Input: part model. Units: mm. Frame: model coordinates. A direction names the side the tool comes from. Give positions to 0.01 mm unless a question says otherwise; leave off trailing zeros. Order: outer loops, then holes, each group sorted by start corner. A loop starts at its lowest first (then second) coordinate and runs counter-clockwise, first axis right, second up. Notation, with made-up numbers: (27.5, -15) -> (43.5, -15) arc R28 cw to (43.5, 3) -> close; hole circle Ø11 at (18, 38). An arc over 180 degrees is marked (long way). Use a Markdown table: item, result. Add a question column.
from build123d import *

# Parameters (mm, degrees)
BOSS_EXTRUDE1_DEPTH = 2
SKETCH3_W           = 2
SKETCH3_H           = 40
SKETCH3_W_2         = 30
SKETCH3_H_2         = 2
BOSS_EXTRUDE2_DEPTH = 3
SKETCH4_R           = 1.75
CUT_EXTRUDE1_DEPTH  = 3
CHAMFER1_SIZE       = 1


with BuildPart() as part:
    # Sketch1 → Boss-Extrude1 (new body)
    with BuildSketch(Plane.XY):
        with BuildLine():
            Line((65.230528188, -85.753133266), (65.230528188, -22.753132266))
            ThreePointArc((65.230528188, -22.753132266), (64.351848531, -20.631811922), (62.230528188, -19.753132266))
            Line((62.230528188, -19.753132266), (-24.769470492, -19.753132266))
            ThreePointArc((-24.769470492, -19.753132266), (-26.890790836, -20.631811922), (-27.769470492, -22.753132266))
            Line((-27.769470492, -22.753132266), (-27.769470492, -85.753133266))
            ThreePointArc((-27.769470492, -85.753133266), (-26.890790836, -87.874453609), (-24.769470492, -88.753133266))
            Line((-24.769470492, -88.753133266), (62.230528188, -88.753133266))
            ThreePointArc((62.230528188, -88.753133266), (64.351848531, -87.874453609), (65.230528188, -85.753133266))
        make_face()
    extrude(amount=BOSS_EXTRUDE1_DEPTH)

    # Sketch3 → Boss-Extrude2 (add)
    with BuildSketch(Plane(origin=(0, 0, 0), x_dir=(-1, 0, 0), z_dir=(0, 0, -1))):
        with Locations((-61.930528188, -54.253132766)):
            Rectangle(SKETCH3_W, SKETCH3_H)
        with Locations((24.469470492, -54.253132766)):
            Rectangle(SKETCH3_W, SKETCH3_H)
        with Locations((-18.730528848, -23.053132266)):
            Rectangle(SKETCH3_W_2, SKETCH3_H_2)
        with Locations((-18.730528848, -85.453133266)):
            Rectangle(SKETCH3_W_2, SKETCH3_H_2)
    extrude(amount=BOSS_EXTRUDE2_DEPTH)

    # Sketch4 → Cut-Extrude1 (cut)
    with BuildSketch(Plane(origin=(0, 0, 0), x_dir=(-1, 0, 0), z_dir=(0, 0, -1))):
        with Locations((-59.230528188, -25.753132266)):
            Circle(SKETCH4_R)
        with Locations((21.769470706, -25.703133912)):
            Circle(SKETCH4_R)
        with Locations((21.769470492, -82.753133266)):
            Circle(SKETCH4_R)
        with Locations((-59.230528188, -82.753133266)):
            Circle(SKETCH4_R)
    extrude(amount=-CUT_EXTRUDE1_DEPTH, mode=Mode.SUBTRACT)

    # Chamfer1
    chamfer1_edges = [part.edges().sort_by_distance(p)[0] for p in [
        (60.980528188, -82.753133266, 2),
        (-20.019470492, -82.753133266, 2),
        (-20.019470706, -25.703133912, 2),
        (60.980528188, -25.753132266, 2),
    ]]
    chamfer(chamfer1_edges, length=CHAMFER1_SIZE)


solid = part.part
Q1. Section query A-A (z = -1.9). Return loops of the section in (x, y).
Q2. Access query for faces 4 (the flat face through (3.731, -85, -1)), 5 (the flat face through (60.931, -55, -1)), 6 (the flat face through (-24, -74.253, -1)), 7 (the flat face through (-24, -34.253, -1)). Directions: +Z, -Z, +X, -X, +Y, -Y. A direction counts if a zero-diameter tool reaches every point of the face in a straight line with its end or side. Return the directions, or none.
Q3. Section query B-B (y = -60). Return loops of the section in (x, z).
Q4. First-contact query: pin 1 (2 mm diameter, centred on x = -24.5, z = -1.5, fed in from +Y); pin 2 (1.5 mm diameter, centred on y = -47.5, z = -1, fed in from +X); pin 3 (2 mm diameter, centred on y = -22.5, z = -1.5, fed in from +X). Flat tips, straight axial feed; report the tip coordinate or a pass-through.
Q5. Draft query along Y for faces 1 (the cylindrical face through (58.423, -84.306, 0.493)), 2 (the flat face through (18, -54, 2)), 3 (the flat face through (18, -88.753, 1)). Return one class per face: +Y half, -Y half, draft (parallel to the pull), parting line (faces both ways), or undercut.
Q6. Section query C-C (x = 22). Return loops of the section in (y, z), plus the area to 3 significant figures.
Q7. Section query D-D (x = 36). Return loops of the section in (y, z), plus the area to 3 significant figures.
Q8. Ray query, line 1 (X direction, y = -59, z = -0.1); line 2 (Y direction, x = 20.5, z = -2.4); line 3 (X direction, y = -26.5, z = 1.4). Return the intervals inside material, ascending.
Solution:
| question | item | result |
|---|---|---|
| 1 | outline | (-25.47, -74.25) -> (-23.47, -74.25) -> (-23.47, -34.25) -> (-25.47, -34.25) -> close; (3.73, -86.45) -> (33.73, -86.45) -> (33.73, -84.45) -> (3.73, -84.45) -> close; (3.73, -24.05) -> (33.73, -24.05) -> (33.73, -22.05) -> (3.73, -22.05) -> close; (60.93, -74.25) -> (62.93, -74.25) -> (62.93, -34.25) -> (60.93, -34.25) -> close |
| 2 | face 4 | -Z, -X, +Y, -Y |
| 2 | face 5 | -Z, +Y, -Y |
| 2 | face 6 | -Z, +X, -X, -Y |
| 2 | face 7 | -Z, +X, -X, +Y |
| 3 | outline | (-27.77, 0) -> (-25.47, 0) -> (-25.47, -3) -> (-23.47, -3) -> (-23.47, 0) -> (60.93, 0) -> (60.93, -3) -> (62.93, -3) -> (62.93, 0) -> (65.23, 0) -> (65.23, 2) -> (-27.77, 2) -> close |
| 4 | pin 1 | stops at y = -34.25 |
| 4 | pin 2 | stops at x = 62.93 |
| 4 | pin 3 | stops at x = 33.73 |
| 5 | face 1 | undercut |
| 5 | face 2 | draft |
| 5 | face 3 | -Y half |
| 6 | outline | (-88.75, 0) -> (-86.45, 0) -> (-86.45, -3) -> (-84.45, -3) -> (-84.45, 0) -> (-24.05, 0) -> (-24.05, -3) -> (-22.05, -3) -> (-22.05, 0) -> (-19.75, 0) -> (-19.75, 2) -> (-88.75, 2) -> close |
| 6 | area | 150 mm² |
| 7 | outline | (-88.75, 0) -> (-19.75, 0) -> (-19.75, 2) -> (-88.75, 2) -> close |
| 7 | area | 138 mm² |
| 8 | line 1 | x = -25.47 to -23.47, 60.93 to 62.93 |
| 8 | line 2 | y = -86.45 to -84.45, -24.05 to -22.05 |
| 8 | line 3 | x = -27.77 to -23.77, -19.77 to 57.21, 61.25 to 65.23 |
